Design review of the part built by this model. Coordinates are the model's own, in mm. Face numbers are marked on the shaded views. A direction names the side the tool comes from. Round coordinates to 2 decimals unless told otherwise and drop trailing zeros. Order: outer loops, then holes, each group sorted by start corner. A loop starts at its lowest first (then second) coordinate and runs counter-clockwise, first axis right, second up.
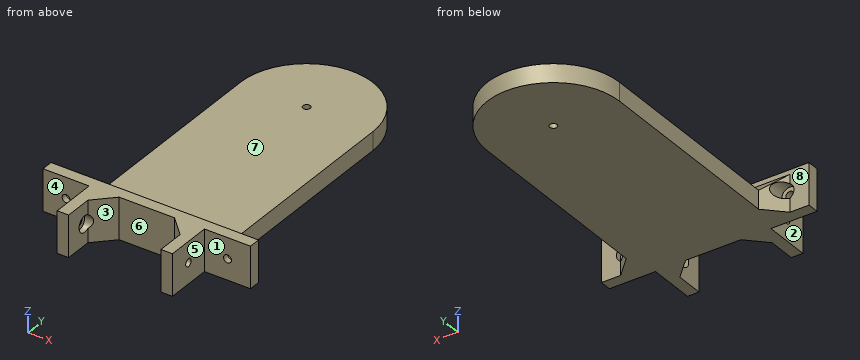
from build123d import *

# Parameters (mm, degrees)
RESSALTO_EXTRUS_O1_DEPTH                     = 8
RESSALTO_EXTRUS_O2_DEPTH                     = 10
CHANFRO1_SIZE                                = 8
ESBO_O3_R                                    = 1.6
CORTE_EXTRUS_O1_DEPTH                        = 138.523416188
REBAIXO_PARA_PARAFUSO_COM_CABE_A_PAN_2_COUNT = 2
REBAIXO_PARA_PARAFUSO_COM_CABE_A_PAN_2_PITCH = 70
CORTE_EXTRUS_O3_REACH                        = 134.856
ESBO_O11_R                                   = 3.5
CORTE_EXTRUS_O4_START                        = 2
ESBO_O19_R                                   = 3.5
CORTE_EXTRUS_O4_DEPTH                        = 2


with BuildPart() as part:
    # Esbo_o1 → Ressalto-extrus_o1 (new body)
    with BuildSketch(Plane.XY):
        with BuildLine():
            Line((28.7, 5), (28.7, 100))
            ThreePointArc((28.7, 100), (0, 128.7), (-28.7, 100))
            Line((-28.7, 100), (-28.7, 5))
            Line((-28.7, 5), (-45, 5))
            Line((-45, 5), (-45, 0))
            Line((-45, 0), (-25, 0))
            Line((-25, 0), (-25, -20))
            Line((-25, -20), (-20, -20))
            Line((-20, -20), (-20, 0))
            Line((-20, 0), (20, 0))
            Line((20, 0), (20, -20))
            Line((20, -20), (25, -20))
            Line((25, -20), (25, 0))
            Line((25, 0), (45, 0))
            Line((45, 0), (45, 5))
            Line((45, 5), (28.7, 5))
        make_face()
    extrude(amount=RESSALTO_EXTRUS_O1_DEPTH)

    # Esbo_o2 → Ressalto-extrus_o2 (add)
    with BuildSketch(Plane.XY.offset(8)):
        Polygon((-20, -20), (-25, -20), (-25, 0), (-45, 0), (-45, 5), (45, 5), (45, 0), (25, 0), (25, -20), (20, -20), (20, 0), (-20, 0), align=None)
    extrude(amount=RESSALTO_EXTRUS_O2_DEPTH)

    # Chanfro1
    chanfro1_edges = [part.edges().sort_by_distance(p)[0] for p in [
        (28.7, 5, 4),
        (20, 0, 9),
        (-20, 0, 9),
        (-28.7, 5, 4),
        (0, 5, 8),
    ]]
    chamfer(chanfro1_edges, length=CHANFRO1_SIZE)

    # Esbo_o3 → Corte-extrus_o1 (cut, through all)
    with BuildSketch(Plane(origin=(0, 0, 0), x_dir=(-1, 0, 0), z_dir=(0, 0, -1))):
        with Locations((0, 100)):
            Circle(ESBO_O3_R)
    extrude(amount=-CORTE_EXTRUS_O1_DEPTH, mode=Mode.SUBTRACT)

    # Esbo_o10 → Rebaixo para parafuso com cabe_a panela (revolve, cut)
    with BuildSketch(Plane(origin=(-35, 5, 9), x_dir=(0, 0, 1), z_dir=(1, 0, 0))):
        Polygon((0, 0), (0, 7.021463052), (1.7, 6), (1.7, 2.4), (3.5, 2.4), (3.5, 0), align=None)
    rebaixo_para_parafuso_com_cabe_a_panela = revolve(axis=Axis((-35, 11.35, 9), (0, -1, 0)), mode=Mode.SUBTRACT)

    # Rebaixo para parafuso com cabe_a pan 2: Rebaixo para parafuso com cabe_a panela ×2
    with Locations(*[(i * REBAIXO_PARA_PARAFUSO_COM_CABE_A_PAN_2_PITCH, 0, 0) for i in range(1, REBAIXO_PARA_PARAFUSO_COM_CABE_A_PAN_2_COUNT)]):
        add(rebaixo_para_parafuso_com_cabe_a_panela, mode=Mode.SUBTRACT)

    # Corte-extrus_o3: up to this face of the body (flat: up to its plane)
    corte_extrus_o3_end = Plane(part.part.faces().sort_by_distance((33.144444444, 8.555555556, 6.222222222))[0])
    # Esbo_o11 → Corte-extrus_o3 (cut, up to the picked face)
    with BuildSketch(Plane(origin=(0, 5, 0), x_dir=(1, 0, 0), z_dir=(0, 1, 0)), mode=Mode.PRIVATE) as corte_extrus_o3_sk1:
        with Locations(Location((35, -9, 0), (0, 0, 270))):
            Circle(ESBO_O11_R)
    corte_extrus_o3_tool1 = split(extrude(corte_extrus_o3_sk1.sketch, amount=CORTE_EXTRUS_O3_REACH, mode=Mode.PRIVATE), bisect_by=corte_extrus_o3_end, keep=Keep.BOTH, mode=Mode.PRIVATE)
    # Esbo_o11 → Corte-extrus_o3 (cut, up to the picked face)
    with BuildSketch(Plane(origin=(0, 5, 0), x_dir=(1, 0, 0), z_dir=(0, 1, 0)), mode=Mode.PRIVATE) as corte_extrus_o3_sk2:
        with Locations(Location((-35, -9, 0), (0, 0, 270))):
            Circle(ESBO_O11_R)
    corte_extrus_o3_tool2 = split(extrude(corte_extrus_o3_sk2.sketch, amount=CORTE_EXTRUS_O3_REACH, mode=Mode.PRIVATE), bisect_by=corte_extrus_o3_end, keep=Keep.BOTH, mode=Mode.PRIVATE)
    add(corte_extrus_o3_tool1.solids().sort_by(Axis((35, 5, 9), (0, 1, 0)))[0], mode=Mode.SUBTRACT)
    add(corte_extrus_o3_tool2.solids().sort_by(Axis((-35, 5, 9), (0, 1, 0)))[0], mode=Mode.SUBTRACT)

    # Esbo_o18 → Rebaixo para parafuso com cabe_a pan 3 (revolve, cut)
    with BuildSketch(Plane(origin=(20, -10, 9), x_dir=(0, 0, 1), z_dir=(0, 1, 0))):
        Polygon((0, 0), (0, 7.021463052), (1.7, 6), (1.7, 2.4), (3.5, 2.4), (3.5, 0), align=None)
    revolve(axis=Axis((13.65, -10, 9), (1, 0, 0)), mode=Mode.SUBTRACT)

    # Esbo_o19 → Corte-extrus_o4 (cut)
    with BuildSketch(Plane.ZY.offset(-20).offset(CORTE_EXTRUS_O4_START)):
        with Locations((9, -10)):
            Circle(ESBO_O19_R)
    corte_extrus_o4 = extrude(amount=-CORTE_EXTRUS_O4_DEPTH, mode=Mode.SUBTRACT)

    # Esbo_o21 → Rebaixo para parafuso com cabe_a pan 4 (revolve, cut)
    with BuildSketch(Plane(origin=(-20, -10, 9), x_dir=(0, 0, -1), z_dir=(0, 1, 0))):
        Polygon((0, 0), (0, 7.021463052), (1.7, 6), (1.7, 2.4), (3.5, 2.4), (3.5, 0), align=None)
    revolve(axis=Axis((-13.65, -10, 9), (-1, 0, 0)), mode=Mode.SUBTRACT)

    # Espelhar1: Corte-extrus_o4 across plane
    add(corte_extrus_o4.mirror(Plane(origin=(0, 0, 0), x_dir=(0, 0, 1), z_dir=(1, 0, 0))), mode=Mode.SUBTRACT)


solid = part.part
1) Take a section at A-A on x = 0. Give the boundary of the cut face in (y, z), plus the area to 3 significant figures.
Results:
outline: (0, 0) - (98.4, 0) - (98.4, 8) - (13, 8) - (5, 16) - (5, 18) - (0, 18) - close; (101.6, 0) - (128.7, 0) - (128.7, 8) - (101.6, 8) - close
area: 1,090 mm2
2) For the marked faces 4, 5, 6, 7 and 8, list the 3-axis set-ups (+Z, -Z, +X, -X, +Y, -Y) from which the entire face can be reached by the end or side of a thin tool; tool diameter is ignored.
Results:
face 4: +Z, -Z, -X, -Y
face 5: +Z, -Z, +X, -Y
face 6: +Z, -Z, -Y
face 7: +Z, +X, -X, +Y
face 8: +Z, +Y
3) Take a section at B-B on z = 3. Give the boundary of the cut face in (x, y), plus the area to 3 significant figures.
Results:
outline: (-45, 0) - (-25, 0) - (-25, -20) - (-20, -20) - (-20, -8) - (-12, 0) - (12, 0) - (20, -8) - (20, -20) - (25, -20) - (25, 0) - (45, 0) - (45, 5) - (36.7, 5) - (28.7, 13) - (28.7, 100) arc R28.7 ccw to (-28.7, 100) - (-28.7, 13) - (-36.7, 5) - (-45, 5) - close; hole circle Ø3.2 at (0, 100)
area: 7,520 mm2
4) Take a section at D-D on x = -35. Give the boundary of the cut face in (y, z), plus the area to 3 significant figures.
Results:
outline: (0, 0) - (6.7, 0) - (6.7, 5.5) - (2.6, 5.5) - (2.6, 7.3) - (0, 7.3) - close; (0, 10.7) - (2.6, 10.7) - (2.6, 12.5) - (6.7, 12.5) - (6.7, 14.3) - (5, 16) - (5, 18) - (0, 18) - close
area: 78.2 mm2
5) To check wall thickness, follow line 1 along X through (y, z) = (1.65, 9); line 2 along Z through (x, y) = (-35, 0.5); line 3 along Y through (x, z) = (24.35, 9). State the ranges of each line that lie inside material, in increasing order.
Results:
line 1: x = -45 to -36.7, -33.3 to 33.3, 36.7 to 45
line 2: z = 0 to 7.3, 10.7 to 18
line 3: y = -20 to -11.7, -8.3 to 12
6) Clearance check with flat-ended pins moving along their axes: P1, Ø8, axis at x = 1, y = 5.5, coming from the -Z side; P2, Ø4.5, axis at x = -35, z = 9, coming from the -Y side; P3, Ø2, axis at y = -10, z = 9, coming from the -X side; P4, Ø3.5, axis at y = -9, z = 10, coming from the +X side. State where each tip first meets the part, or that it passes through.
Results:
P1: stops at z = 0
P2: stops at y = 0
P3: passes through
P4: stops at x = 25
7) The part is to be moulded in two halves that separate along X. For the marked faces 1, 2 and 3, say which applies: released by +X, released by -X, zero draft, split by the parting line, or undercut.
Results:
face 1: zero draft
face 2: released by -X
face 3: undercut
8) Take a section at C-C on z = 14.25. Give the boundary of the cut face in (x, y), plus the area to 3 significant figures.
Results:
outline: (-45, 0) - (-25, 0) - (-25, -20) - (-20, -20) - (-20, -8) - (-12, 0) - (12, 0) - (20, -8) - (20, -20) - (25, -20) - (25, 0) - (45, 0) - (45, 5) - (36.7, 5) - (34.95, 6.75) - (-34.95, 6.75) - (-36.7, 5) - (-45, 5) - close
area: 839 mm2
